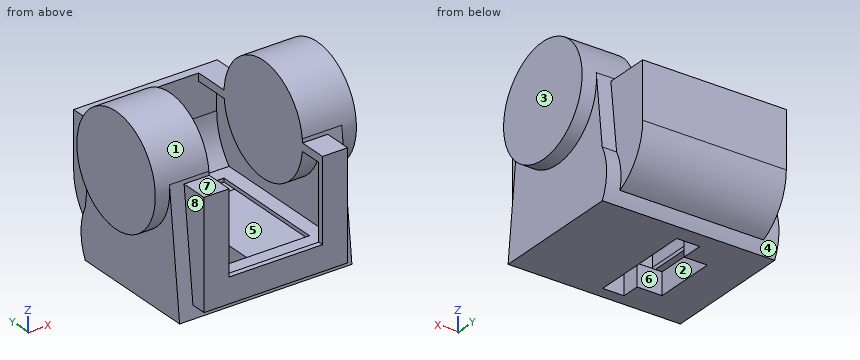
```python
from build123d import *

# Parameters (mm, degrees)
F1_DEPTH  = 76.2
F2_R      = 48.462003
F3_DEPTH  = 88.9
F5_DEPTH  = 63.5
F7_DEPTH  = 41.275
F9_DEPTH  = 57.15
F11_W     = 122.617453
F11_H     = 143.214412
F11_W_2   = 87.062612
F11_H_2   = 105.60561
F12_DEPTH = 3.302
F14_DEPTH = 25.4


with BuildPart() as f1:
    # F0 (on Right) → F1 (new body, symmetric)
    with BuildSketch(Plane.YZ):
        with BuildLine():
            Line((-45.672867, 108.644605), (-58.206145, 0))
            Line((-58.206145, 0), (58.235409, 0))
            ThreePointArc((58.235409, 0), (63.473631, 22.12486), (58.046448, 44.204128))
            Line((58.046448, 44.204128), (50.612573, 108.644605))
            ThreePointArc((50.612573, 108.644605), (2.469853, 151.552848), (-45.672867, 108.644605))
        make_face()
    extrude(amount=F1_DEPTH, both=True)

    # F2 (on Right) → F3 (join, symmetric)
    with BuildSketch(Plane.YZ):
        with Locations((2.469853, 103.090845)):
            Circle(F2_R)
    extrude(amount=F3_DEPTH, both=True)

    # F4 (on Right) → F5 (join, symmetric)
    with BuildSketch(Plane.YZ):
        with BuildLine():
            Line((90.254351, 105.402268), (-70.632874, 105.402268))
            Line((-70.632874, 105.402268), (-70.632874, 10.851024))
            Line((-70.632874, 10.851024), (62.193779, 10.851024))
            ThreePointArc((62.193779, 10.851024), (82.663095, 29.299382), (90.254351, 55.789147))
            Line((90.254351, 55.789147), (90.254351, 105.402268))
        make_face()
    extrude(amount=F5_DEPTH, both=True)

    # F6 (on Right) → F7 (cut, symmetric)
    with BuildSketch(Plane.YZ):
        with BuildLine():
            Line((82.148224, 166.311592), (-101.252101, 166.311592))
            Line((-101.252101, 166.311592), (-101.252101, 32.949033))
            Line((-101.252101, 32.949033), (-65.976813, 32.949033))
            Line((-65.976813, 32.949033), (-65.976813, 19.525689))
            Line((-65.976813, 19.525689), (52.960247, 19.525689))
            ThreePointArc((52.960247, 19.525689), (74.312895, 40.444956), (82.148224, 69.292121))
            Line((82.148224, 69.292121), (82.148224, 166.311592))
        make_face()
    extrude(amount=F7_DEPTH, both=True, mode=Mode.SUBTRACT)

    # F8 (on Right) → F9 (cut, symmetric)
    with BuildSketch(Plane.YZ):
        with BuildLine():
            ThreePointArc((50.721201, 98.577179), (2.53727, 54.628888), (-45.76875, 98.442949))
            Line((-45.76875, 98.442949), (-65.976813, 98.442949))
            Line((-65.976813, 98.442949), (-65.976813, 19.525689))
            Line((-65.976813, 19.525689), (52.960247, 19.525689))
            ThreePointArc((52.960247, 19.525689), (74.312895, 40.444956), (82.148224, 69.292121))
            Line((82.148224, 69.292121), (82.148224, 98.577179))
            Line((82.148224, 98.577179), (50.721201, 98.577179))
        make_face()
    extrude(amount=F9_DEPTH, both=True, mode=Mode.SUBTRACT)

    # F11 (on offset) → F12 (join)
    with BuildSketch(Plane.XY.offset(30.48)):
        with Locations((-0.147897, 3.422026)):
            Rectangle(F11_W, F11_H)
        with Locations((0.489652, 2.055012)):
            Rectangle(F11_W_2, F11_H_2, mode=Mode.SUBTRACT)
    extrude(amount=-F12_DEPTH)

    # F13 (on Top) → F14 (cut)
    with BuildSketch(Plane.XY):
        Polygon((-40.871959, 24.293846), (-40.871959, -31.535055), (-18.801486, -31.535055), (-18.801486, -47.650613), (0, -47.650613), (0, 43.670883), (-20.343806, 43.670883), (-20.343806, 24.293846), align=None)
    extrude(amount=F14_DEPTH, mode=Mode.SUBTRACT)


solid = f1.part
```
Read the model definition and answer for the solid it produces. Units are mm, in the model's axes. Face numbers are marked on the shaded views. A direction names the side the tool comes from. Coordinates: 2 decimals unless noted, no trailing zeros. Order: outer loops, then holes, each group sorted by start corner. A loop starts at its lowest first (then second) coordinate and runs counter-clockwise, first axis right, second up. Notation, with made-up numbers: (60, 21.25) - (67, 21.25) arc R25 ccw to (67, 35.25) - close; hole circle Ø4 at (52, 67.25). An arc over 180 degrees is marked (long way). Answer as a JSON object with one key per item and string values. Group by question number.
Item 1: Section A-A (y = 17) is taken. Give the vertices of the cut face in (x, z) (3 decimals).
Item 2: Flat-ended cylindrical pins translate along their axes: P1, Ø1.5, axis at x = 19.5, y = -49.5, coming from the +Z side; P2, Ø11, axis at x = 10, y = -66.5, coming from the -Z side; P3, Ø8, axis at x = 54.5, y = 11, coming from the +Z side. Find the tip coordinate at first contact, or state that the pin passes through.
Item 3: A tool of negligible diameter and unlimited length cuts with its end or side. For the marked faces 4, 5, 6, 7 and 8, from which of +Z, -Z, +X, -X, +Y, -Y can it reach the whole face along a straight path? Write none if from no direction.
Item 4: Section B-B (x = 3) is taken. Give the vertices of the cut face in (y, z), plus the area to 3 significant figures.
Item 5: Section D-D (z = 137) is taken. Give the vertices of the cut face in (x, y) (3 decimals), plus the area to 3 significant figures.
Item 6: Consider probe 1 along X at (y, z) = (41.5, 91.5) (3 decimals); probe 2 along X at (y, z) = (9, 10.5); probe 3 along Z at (x, y) = (-57, -16.5). Determine where each line is inside the solid, lowest interval first. Write a range as from..to.
Item 7: The mould has two halves that part along Y. Classify the marked faces 1, 2 and 3: +Y half, -Y half, draft (parallel to the pull), parting line (faces both ways), or undercut.
Item 8: Section C-C (z = 22) is taken. Give the vertices of the cut face in (x, y), plus the area to 3 significant figures.
Results are:
{
 "1": {"outline": "(-88.9, 56.858) - (-76.2, 56.858) - (-76.2, 0) - (-40.872, 0) - (-40.872, 19.526) - (-57.15, 19.526) - (-57.15, 27.178) - (-43.042, 27.178) - (-43.042, 30.48) - (-57.15, 30.48) - (-57.15, 56.858) - (-41.275, 56.858) - (-41.275, 149.323) - (-88.9, 149.323) - close; (0, 0) - (76.2, 0) - (76.2, 56.858) - (88.9, 56.858) - (88.9, 149.323) - (41.275, 149.323) - (41.275, 56.858) - (57.15, 56.858) - (57.15, 30.48) - (44.021, 30.48) - (44.021, 27.178) - (57.15, 27.178) - (57.15, 19.526) - (0, 19.526) - close"},
 "2": {"P1": "stops at z = 19.53", "P2": "stops at z = 10.85", "P3": "stops at z = 151.34"},
 "3": {"face 4": "+Y", "face 5": "none", "face 6": "+Z, -Z", "face 7": "+Z, +X, -X, -Y", "face 8": "+Z, -X, -Y"},
 "4": {"outline": "(-70.63, 10.85) - (-56.95, 10.85) - (-58.21, 0) - (58.24, 0) arc R48.47 ccw to (62.19, 10.85) arc R50.01 ccw to (90.25, 55.79) - (90.25, 105.4) - (82.15, 105.4) - (82.15, 69.29) arc R57.02 cw to (66.9, 30.48) - (54.86, 30.48) - (54.86, 27.18) - (63.57, 27.18) arc R57.02 cw to (52.96, 19.53) - (-65.98, 19.53) - (-65.98, 27.18) - (-50.75, 27.18) - (-50.75, 30.48) - (-65.98, 30.48) - (-65.98, 32.95) - (-70.63, 32.95) - close", "area": "3,580 mm^2"},
 "5": {"outline": "(-88.9, -32.153) - (-41.275, -32.153) - (-41.275, 37.093) - (-88.9, 37.093) - close; (41.275, -32.153) - (88.9, -32.153) - (88.9, 37.093) - (41.275, 37.093) - close", "area": "6,600 mm^2"},
 "6": {"probe 1": "x = -88.9..-41.275, 41.275..88.9", "probe 2": "x = -76.2..-40.87, 0..76.2", "probe 3": "z = 0..19.53, 27.18..30.48, 58.5..147.69"},
 "7": {"face 1": "parting line", "face 2": "undercut", "face 3": "draft"},
 "8": {"outline": "(-76.2, -55.67) - (-63.5, -55.67) - (-63.5, -70.63) - (63.5, -70.63) - (63.5, -55.67) - (76.2, -55.67) - (76.2, 63.47) - (63.5, 63.47) - (63.5, 77.11) - (-63.5, 77.11) - (-63.5, 63.47) - (-76.2, 63.47) - close; hole (-57.15, -65.98) - (57.15, -65.98) - (57.15, 56.98) - (-57.15, 56.98) - close", "area": "7,740 mm^2"}
}
